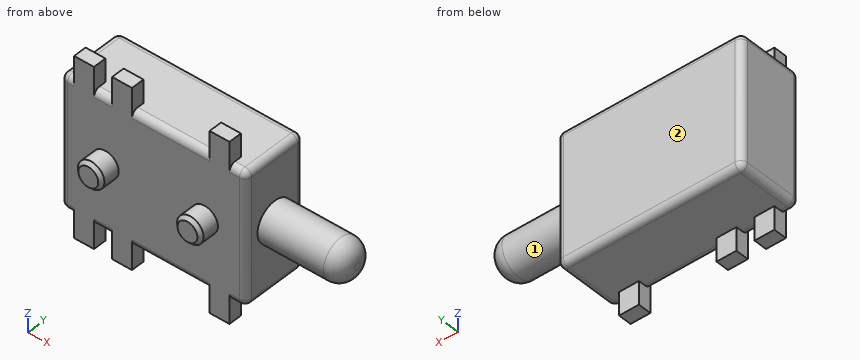
from build123d import *

# Parameters (mm, degrees)
SKETCH_1_W      = 5.6
SKETCH_1_H      = 4
EXTRUDE_1_DEPTH = 2
SKETCH_2_R      = 0.6
EXTRUDE_2_DEPTH = 2.5
FILLET_1_R      = 0.5
SKETCH_3_W      = 0.6
SKETCH_3_H      = 5.4
EXTRUDE_3_DEPTH = 0.4
SKETCH_4_R      = 0.4
EXTRUDE_4_DEPTH = 0.6
CHAMFER_1_SIZE  = 0.1
FILLET_2_R      = 0.2


with BuildPart() as part:
    # Эскиз1 → Бобышка-Вытянуть1 (new body)
    with BuildSketch(Plane(origin=(0, 0, 0), x_dir=(1, 0, 0), z_dir=(0, 1, 0))):
        Rectangle(SKETCH_1_W, SKETCH_1_H)
    extrude(amount=EXTRUDE_1_DEPTH)

    # Эскиз2 → Бобышка-Вытянуть2 (add)
    with BuildSketch(Plane(origin=(2.8, 0, 0), x_dir=(0, 0, -1), z_dir=(1, 0, 0))):
        with Locations((0, 1)):
            Circle(SKETCH_2_R)
    extrude(amount=EXTRUDE_2_DEPTH)

    # Скругление1
    fillet_1_edges = [part.edges().sort_by_distance(p)[0] for p in [
        (5.3, 1, 0.6),
    ]]
    fillet(fillet_1_edges, radius=FILLET_1_R)

    # Эскиз3 → Бобышка-Вытянуть3 (add)
    with BuildSketch(Plane.XZ):
        with Locations((-2.1, 0)):
            Rectangle(SKETCH_3_W, SKETCH_3_H)
        with Locations((-0.95, 0)):
            Rectangle(SKETCH_3_W, SKETCH_3_H)
        with Locations((2, 0)):
            Rectangle(SKETCH_3_W, SKETCH_3_H)
    extrude(amount=-EXTRUDE_3_DEPTH)

    # Эскиз4 → Бобышка-Вытянуть4 (add)
    with BuildSketch(Plane.XZ):
        with Locations((-1.45, 0)):
            Circle(SKETCH_4_R)
        with Locations((1.55, 0)):
            Circle(SKETCH_4_R)
    extrude(amount=EXTRUDE_4_DEPTH)

    # Фаска1
    chamfer_1_edges = [part.edges().sort_by_distance(p)[0] for p in [
        (-1.85, -0.6, 0),
        (1.15, -0.6, 0),
    ]]
    chamfer(chamfer_1_edges, length=CHAMFER_1_SIZE)

    # Скругление2
    fillet_2_edges = [part.edges().sort_by_distance(p)[0] for p in [
        (-2.8, 2, 0),
        (0, 2, 2),
        (-1.525, 0, 2),
        (-2.6, 0, -2),
        (2.8, 2, 0),
        (-1.525, 0, -2),
        (0.525, 0, 2),
        (-2.6, 0, 2),
        (-2.8, 0, 0),
        (2.55, 0, -2),
        (2.8, 0, 0),
        (0.525, 0, -2),
        (2.55, 0, 2),
        (0, 2, -2),
        (2.8, 1, 2),
        (-2.8, 1, 2),
        (-2.8, 1, -2),
        (2.8, 1, -2),
    ]]
    fillet(fillet_2_edges, radius=FILLET_2_R)


solid = part.part
For this review, take the finished solid that the model builds, in its own axes (mm). Face numbers are marked on the shaded views. A direction names the side the tool comes from. Round coordinates to 2 decimals unless told otherwise and drop trailing zeros. Order: outer loops, then holes, each group sorted by start corner. A loop starts at its lowest first (then second) coordinate and runs counter-clockwise, first axis right, second up. Notation, with made-up numbers: (33, 80) -> (60, 80) arc R18 ccw to (60, 114) -> close; hole circle Ø1 at (0, 30.5). An arc over 180 degrees is marked (long way). Put each result on its own line as item: value.
Q1. Add section B-B on z = -1.15. Write out the cut boundary in (x, y).
Check result:
outline: (-2.8, 0.2) arc R0.2 ccw to (-2.6, 0) -> (2.6, 0) arc R0.2 ccw to (2.8, 0.2) -> (2.8, 1.8) arc R0.2 ccw to (2.6, 2) -> (-2.6, 2) arc R0.2 ccw to (-2.8, 1.8) -> close
Q2. Add section A-A on x = -1.45. Write out the cut boundary in (y, z), plus the area to 3 significant figures.
Check result:
outline: (-0.6, -0.3) -> (-0.5, -0.4) -> (0, -0.4) -> (0, -1.8) arc R0.2 ccw to (0.2, -2) -> (1.8, -2) arc R0.2 ccw to (2, -1.8) -> (2, 1.8) arc R0.2 ccw to (1.8, 2) -> (0.2, 2) arc R0.2 ccw to (0, 1.8) -> (0, 0.4) -> (-0.5, 0.4) -> (-0.6, 0.3) -> close
area: 8.44 mm2
Q3. Insertion check: pin 1 Ø1 at (x, z) = (-1, 1.5) entering from -Y; pin 2 Ø1 at (y, z) = (0.5, -0.5) entering from +X. Each pin has a flat end and moves straight along its axis. Give the tip position at first contact, or say it passes through.
Check result:
pin 1: y = 0
pin 2: x = 5.29
Q4. For probe 1 along Y at (x, z) = (-2, -0.4); probe 2 along Z at (x, y) = (1.5, 1.3); probe 3 along X at (y, z) = (0.3, 0.5), list the stretches that pass through material, from the lowest coordinate up. Write a range as [from, to].
Check result:
probe 1: [0, 2]
probe 2: [-2, 2]
probe 3: [-2.8, 2.8]
Q5. Add section D-D on x = 3.75. Write out the cut boundary in (y, z), plus the area to 3 significant figures.
Check result:
outline: circle Ø1.2 at (1, 0)
area: 1.13 mm2
Q6. Machinability: for the marked faces 1 and 2, which of the approach directions +Z, -Z, +X, -X, +Y, -Y give a long, thin tool a straight path to every point of the face, cutting with its end or side? Answer none if there is none.
Check result:
face 1: +X
face 2: +Z, -Z, +X, -X, +Y
